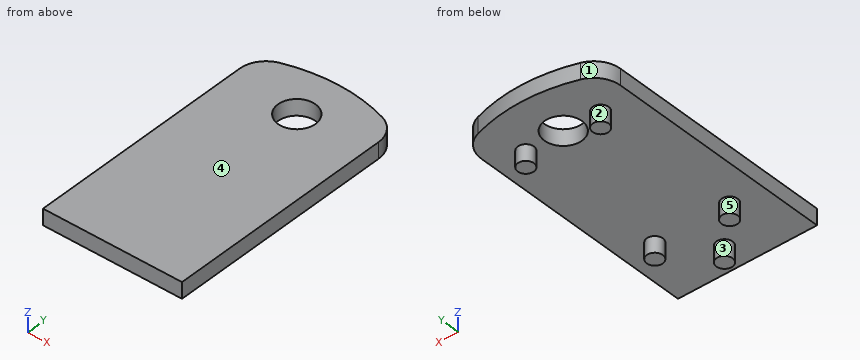
Autodesk Inventor part; units mm, degrees
ref_plane "YZ Plane" through (0, 0, 0) normal (1, 0, 0) x (0, 1, 0)
ref_plane "XZ Plane" through (0, 0, 0) normal (0, 1, 0) x (-1, 0, 0)
ref_plane "XY Plane" through (0, 0, 0) normal (0, 0, 1) x (1, 0, 0)
sketch "Эскиз1" plane through (0, 0, 0) normal (0, 0, 1) x (1, 0, 0)
  circle A0 centre (-7, 12) radius 1.5
  circle A1 centre (0, 5) radius 1.5
  circle A2 centre (7, 12) radius 1.5
  circle A3 centre (7, 40) radius 1.5
  circle A4 centre (-7, 40) radius 1.5
  point P0 (0, 0)
extrude "Выдавливание1" add sketch "Эскиз1" against normal blind 3
sketch "Эскиз3" plane through (0, 5, 0) normal (0, 0, 1) x (1, 0, 0)
  line L0 (-13, -5) -> (-13, 37.6484)
  line L1 (13, 37.6484) -> (13, -5)
  line L2 (13, -5) -> (-13, -5)
  circle A0 centre (0, 35) radius 3.5
  arc A1 (13, 37.6484) -> (9.6, 42.3855) centre (8, 37.6484) ccw
  arc A2 (9.6, 42.3855) -> (-9.6, 42.3855) centre (0, 13.963) ccw
  arc A3 (-9.6, 42.3855) -> (-13, 37.6484) centre (-8, 37.6484) ccw
  point P0 (0, -5)
extrude "Выдавливание2" add sketch "Эскиз3" along normal blind 3
properties part number "gasket_2"
Model file for the job. Use its own axes, mm. Face numbers are marked on the shaded views. A direction names the side the tool comes from. Give positions to 0.01 mm unless a question says otherwise; leave off trailing zeros. Loops run counter-clockwise (first coordinate to the right, second up) from the corner with the lowest first, then second, coordinate; pieces in that order, holes last. Notation, with made-up numbers: (-39.5, 18.5) -> (-33.5, 18.5) arc R32 ccw to (-33.5, 48.5) -> close; hole circle Ø11 at (48, 41). An arc over 180 degrees is marked (long way). Use CSV: the item, a comma, the result in double quotes. Start each with the question number.
1) Slice it at B-B on z = 0.5. Give the cut face in (x, y), plus the area to 3 significant figures.
2) Tool access for the marked faces 1 and 2: list every direction of +Z, -Z, +X, -X, +Y, -Y with a clear straight run to the whole face (end or side of a thin tool).
3) Mould opens along X. For the marked faces 3, 4 and 5 say: released by +X, released by -X, zero draft, split by the parting line, or undercut.
4) Slice it at C-C on x = 0. Give the cut face in (y, z).
5) Slice it at A-A on y = 40. Give the cut face in (x, z).
6) Flat gauge pins, fed straight in: pin 1 Ø8 at (x, y) = (-1.5, 28) entering from -Z; pin 2 Ø6.5 at (x, y) = (0, 40) entering from +Z. Where does each tip first touch, or does it go through?
7) Wall check: line 1 (Z direction, x = -4, y = 23); line 2 (X direction, y = 11, z = -2.05); line 3 (Y direction, x = -8.25, z = -1.4). Give the ranges that are in metal, low to high.
8) Slice it at D-D on y = 5. Give the cut face in (x, z), plus the area to 3 significant figures.
Computed values:
1,outline,"(-13, 0) -> (13, 0) -> (13, 42.65) arc R5 ccw to (9.6, 47.39) arc R30 ccw to (-9.6, 47.39) arc R5 ccw to (-13, 42.65) -> close; hole circle Ø7 at (0, 40)"
1,area,"1,210 mm^2"
2,face 1,"+Z, -Z, -X, +Y"
2,face 2,"-Z"
3,face 3,"split by the parting line"
3,face 4,"zero draft"
3,face 5,"undercut"
4,outline,"(0, 0) -> (3.5, 0) -> (3.5, -3) -> (6.5, -3) -> (6.5, 0) -> (36.5, 0) -> (36.5, 3) -> (0, 3) -> close; (43.5, 0) -> (48.96, 0) -> (48.96, 3) -> (43.5, 3) -> close"
5,outline,"(-13, 0) -> (-8.5, 0) -> (-8.5, -3) -> (-5.5, -3) -> (-5.5, 0) -> (-3.5, 0) -> (-3.5, 3) -> (-13, 3) -> close; (3.5, 0) -> (5.5, 0) -> (5.5, -3) -> (8.5, -3) -> (8.5, 0) -> (13, 0) -> (13, 3) -> (3.5, 3) -> close"
6,pin 1,"stops at z = 0"
6,pin 2,"passes through"
7,line 1,"z = 0 to 3"
7,line 2,"x = -8.12 to -5.88, 5.88 to 8.12"
7,line 3,"y = 11.17 to 12.83, 39.17 to 40.83"
8,outline,"(-13, 0) -> (-1.5, 0) -> (-1.5, -3) -> (1.5, -3) -> (1.5, 0) -> (13, 0) -> (13, 3) -> (-13, 3) -> close"
8,area,"87.0 mm^2"
